Here's how the part is built. I have some questions about the finished solid (model axes, mm). Give positions to 0.01 mm unless a question says otherwise; leave off trailing zeros. Loops run counter-clockwise (first coordinate to the right, second up) from the corner with the lowest first, then second, coordinate; pieces in that order, holes last. Notation, with made-up numbers: (-37, 40.25) - (-24, 40.25) arc R28 cw to (-24, 77.25) - close; hole circle Ø4 at (24.25, -2.5). An arc over 180 degrees is marked (long way). Use one line per item in the form item = value.
from build123d import *

# Parameters (mm, degrees)
F0_R     = 44.45
F0_R_2   = 41.91
F1_DEPTH = 25.4
F2_R     = 41.91
F2_R_2   = 38.1
F3_DEPTH = 5.08
F4_R     = 5.08
F5_DEPTH = 56.642


with BuildPart() as f1:
    # F0 (on Top) → F1 (new body)
    with BuildSketch(Plane.XY):
        Circle(F0_R)
        Circle(F0_R_2, mode=Mode.SUBTRACT)
    extrude(amount=F1_DEPTH)

    # F2 (on face) → F3 (join)
    with BuildSketch(Plane.XY.offset(25.4)):
        Circle(F2_R)
        Circle(F2_R_2, mode=Mode.SUBTRACT)
        Circle(F2_R_2)
    extrude(amount=-F3_DEPTH)

    # F4 (on Front) → F5 (cut, symmetric)
    with BuildSketch(Plane.XZ):
        with Locations((0, 7.133455)):
            Circle(F4_R)
    extrude(amount=F5_DEPTH, both=True, mode=Mode.SUBTRACT)


solid = f1.part
(1) If we section it at D-D (z = 16.5): List the corners of the cut face in (x, y) for me, plus the area to 3 significant figures.
Geometry says:
outline = circle Ø88.9 at (0, 0); hole circle Ø83.82 at (0, 0)
area = 689 mm²
(2) If we section it at A-A (x = 0): List the corners of the cut face in (y, z) for me, plus the area to 3 significant figures.
Geometry says:
outline = (-44.45, 0) - (-41.91, 0) - (-41.91, 2.05) - (-44.45, 2.05) - close; (-44.45, 12.21) - (-41.91, 12.21) - (-41.91, 20.32) - (41.91, 20.32) - (41.91, 12.21) - (44.45, 12.21) - (44.45, 25.4) - (-44.45, 25.4) - close; (41.91, 0) - (44.45, 0) - (44.45, 2.05) - (41.91, 2.05) - close
area = 503 mm²
(3) If I drill on probe 1 along Y at (x, z) = (0, 16); probe 2 along X at (y, z) = (-1, 20.25); probe 3 along Z at (x, y) = (0, 42.4), over which ranges is the centre line in solid material (lowest first)?
Geometry says:
probe_1 = -44.45 to -41.91, 41.91 to 44.45
probe_2 = -44.44 to -41.9, 41.9 to 44.44
probe_3 = 0 to 2.05, 12.21 to 25.4
(4) If we section it at B-B (y = 0): List the corners of the cut face in (x, z) for me.
Geometry says:
outline = (-44.45, 0) - (-41.91, 0) - (-41.91, 20.32) - (41.91, 20.32) - (41.91, 0) - (44.45, 0) - (44.45, 25.4) - (-44.45, 25.4) - close
(5) For P1, Ø6, axis at y = 29.5, z = 5, coming from the +X side; P2, Ø10, axis at y = -23.5, z = 12, coming from the -X side; P3, Ø3, axis at x = 11, y = -3, coming from the -Z side, each with a flat end and sliding along its axis, tell me the tip position at first contact or that it passes through.
Geometry says:
P1 = 35.69
P2 = -40.42
P3 = 20.32
(6) Thinking about a two-plate mould opening in Y: for faces 1 (the cylindrical face through (-5.456, 41.553, 10.018)), 2 (the flat face through (-1, 1, 20.32)), 3 (the flat face through (-1, 1, 25.4)), 4 (the cylindrical face through (42.397, 13.352, 12.522)), which applies, pulls with the +Y half, pulls with the -Y half, needs draft (parallel to the pull), parting line crosses it, or undercut?
Geometry says:
face_1 = undercut
face_2 = undercut
face_3 = needs draft
face_4 = parting line crosses it
